Geometry check sheet. Reference: the model listing, model coordinates, mm. Give positions to 0.01 mm unless a question says otherwise; leave off trailing zeros. Loops run counter-clockwise (first coordinate to the right, second up) from the corner with the lowest first, then second, coordinate; pieces in that order, holes last. Notation, with made-up numbers: (20, 7.25) - (64, 7.25) arc R25 ccw to (64, 19.25) - close; hole circle Ø10 at (2.5, 52). An arc over 180 degrees is marked (long way). Use a Markdown table: item, result. Add a question column.
1. Cross-section at A-A on z = 160. Enter the section's corners in (x, y) (3 decimals).
2. Cross-section at C-C on x = 580. Enter the section's corners in (y, z) (3 decimals).
3. Cross-section at B-B on y = -74. Enter the section's corners in (x, z) (3 decimals).
4. Material ranges on L1, parallel to X at y = -20.5, z = 1498.5 (3 decimals); L2, parallel to X at y = -2, z = 38 (3 decimals); L3, parallel to Z at x = 1028, y = -17.5 (3 decimals), recorded low to high.
5. Depth check by flat-ended pin: P1, Ø1.6, axis at x = 1539, y = -1.5, coming from the -Z side; P2, Ø3.5, axis at y = -2.5, z = 1845, coming from the +X side; P3, Ø2, axis at y = -46, z = 357, coming from the -X side. Enter the tip coordinate at first touch or a pass-through.
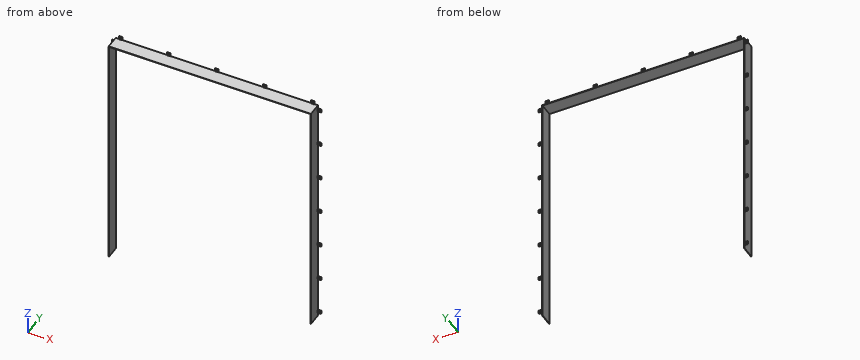
from build123d import *

# Parameters (mm, degrees)
F1_DEPTH = 101.6
F0_W     = 25.4
F0_H     = 25.4
F0_R     = 3.81
F2_DEPTH = 3.175


# Not quite as in the source:
# - a feature names something its author has since deleted; it is built from what else it names


with BuildPart() as f1:
    # F0 (on Front) → F1 (new body)
    with BuildSketch(Plane.XZ):
        Polygon((0, 25.4), (0, 0), (3.175, 0), (3.175, 1828.8), (1527.175, 1828.8), (1527.175, 0), (1530.35, 0), (1530.35, 25.4), (1530.35, 50.8), (1530.35, 318.0291666667), (1530.35, 343.4291666667), (1530.35, 610.6583333333), (1530.35, 636.0583333333), (1530.35, 903.2875), (1530.35, 928.6875), (1530.35, 1195.9166666667), (1530.35, 1221.3166666667), (1530.35, 1488.5458333333), (1530.35, 1513.9458333333), (1530.35, 1781.175), (1530.35, 1806.575), (1530.35, 1831.975), (1504.95, 1831.975), (1479.55, 1831.975), (1141.4125, 1831.975), (1116.0125, 1831.975), (777.875, 1831.975), (752.475, 1831.975), (414.3375, 1831.975), (388.9375, 1831.975), (50.8, 1831.975), (25.4, 1831.975), (0, 1831.975), (0, 1806.575), (0, 1781.175), (0, 1513.9458333333), (0, 1488.5458333333), (0, 1221.3166666667), (0, 1195.9166666667), (0, 928.6875), (0, 903.2875), (0, 636.0583333333), (0, 610.6583333333), (0, 343.4291666667), (0, 318.0291666667), (0, 50.8), align=None)
    extrude(amount=F1_DEPTH)

    # F0 (on Front) → F2 (join)
    with BuildSketch(Plane.XZ):
        with Locations((-12.7, 38.1)):
            Rectangle(F0_W, F0_H)
        with Locations((-12.7, 38.1)):
            Circle(F0_R, mode=Mode.SUBTRACT)
        with Locations((-12.7, 330.7291666667)):
            Rectangle(F0_W, F0_H)
        with Locations((-12.7, 330.7291666667)):
            Circle(F0_R, mode=Mode.SUBTRACT)
        with Locations((-12.7, 623.3583333333)):
            Rectangle(F0_W, F0_H)
        with Locations((-12.7, 623.3583333333)):
            Circle(F0_R, mode=Mode.SUBTRACT)
        with Locations((1543.05, 38.1)):
            Rectangle(F0_W, F0_H)
        with Locations((1543.05, 38.1)):
            Circle(F0_R, mode=Mode.SUBTRACT)
        with Locations((-12.7, 915.9875)):
            Rectangle(F0_W, F0_H)
        with Locations((-12.7, 915.9875)):
            Circle(F0_R, mode=Mode.SUBTRACT)
        with Locations((1543.05, 330.7291666667)):
            Rectangle(F0_W, F0_H)
        with Locations((1543.05, 330.7291666667)):
            Circle(F0_R, mode=Mode.SUBTRACT)
        with Locations((-12.7, 1208.6166666667)):
            Rectangle(F0_W, F0_H)
        with Locations((-12.7, 1208.6166666667)):
            Circle(F0_R, mode=Mode.SUBTRACT)
        with Locations((1543.05, 623.3583333333)):
            Rectangle(F0_W, F0_H)
        with Locations((1543.05, 623.3583333333)):
            Circle(F0_R, mode=Mode.SUBTRACT)
        with Locations((-12.7, 1501.2458333333)):
            Rectangle(F0_W, F0_H)
        with Locations((-12.7, 1501.2458333333)):
            Circle(F0_R, mode=Mode.SUBTRACT)
        with Locations((1543.05, 915.9875)):
            Rectangle(F0_W, F0_H)
        with Locations((1543.05, 915.9875)):
            Circle(F0_R, mode=Mode.SUBTRACT)
        with Locations((-12.7, 1793.875)):
            Rectangle(F0_W, F0_H)
        with Locations((-12.7, 1793.875)):
            Circle(F0_R, mode=Mode.SUBTRACT)
        with Locations((1543.05, 1208.6166666667)):
            Rectangle(F0_W, F0_H)
        with Locations((1543.05, 1208.6166666667)):
            Circle(F0_R, mode=Mode.SUBTRACT)
        with Locations((38.1, 1844.675)):
            Rectangle(F0_W, F0_H)
        with Locations((38.1, 1844.675)):
            Circle(F0_R, mode=Mode.SUBTRACT)
        with Locations((1543.05, 1501.2458333333)):
            Rectangle(F0_W, F0_H)
        with Locations((1543.05, 1501.2458333333)):
            Circle(F0_R, mode=Mode.SUBTRACT)
        with Locations((401.6375, 1844.675)):
            Rectangle(F0_W, F0_H)
        with Locations((401.6375, 1844.675)):
            Circle(F0_R, mode=Mode.SUBTRACT)
        with Locations((1543.05, 1793.875)):
            Rectangle(F0_W, F0_H)
        with Locations((1543.05, 1793.875)):
            Circle(F0_R, mode=Mode.SUBTRACT)
        with Locations((765.175, 1844.675)):
            Rectangle(F0_W, F0_H)
        with Locations((765.175, 1844.675)):
            Circle(F0_R, mode=Mode.SUBTRACT)
        with Locations((1492.25, 1844.675)):
            Rectangle(F0_W, F0_H)
        with Locations((1492.25, 1844.675)):
            Circle(F0_R, mode=Mode.SUBTRACT)
        with Locations((1128.7125, 1844.675)):
            Rectangle(F0_W, F0_H)
        with Locations((1128.7125, 1844.675)):
            Circle(F0_R, mode=Mode.SUBTRACT)
    extrude(amount=F2_DEPTH)


solid = f1.part
Values found:
| question | item | result |
|---|---|---|
| 1 | outline | (0, -101.6) - (3.175, -101.6) - (3.175, 0) - (0, 0) - close; (1527.175, -101.6) - (1530.35, -101.6) - (1530.35, 0) - (1527.175, 0) - close |
| 2 | outline | (-101.6, 1828.8) - (0, 1828.8) - (0, 1831.975) - (-101.6, 1831.975) - close |
| 3 | outline | (0, 0) - (3.175, 0) - (3.175, 1828.8) - (1527.175, 1828.8) - (1527.175, 0) - (1530.35, 0) - (1530.35, 1831.975) - (0, 1831.975) - close |
| 4 | L1 | x = 0 to 3.175, 1527.175 to 1530.35 |
| 4 | L2 | x = -25.4 to -16.509, -8.891 to 3.175, 1527.175 to 1539.241, 1546.859 to 1555.75 |
| 4 | L3 | z = 1828.8 to 1831.975 |
| 5 | P1 | stops at z = 25.4 |
| 5 | P2 | stops at x = 1504.95 |
| 5 | P3 | stops at x = 0 |
